Check sheet for the modelled part. Datum: model origin and axes. Units: mm. A direction names the side the tool comes from. Round coordinates to 2 decimals unless told otherwise and drop trailing zeros. Loops run counter-clockwise (first coordinate to the right, second up) from the corner with the lowest first, then second, coordinate; pieces in that order, holes last. Notation, with made-up numbers: (43, 16.5) -> (75, 16.5) arc R22 cw to (75, 38.5) -> close; hole circle Ø4 at (23.5, 61.5). An arc over 180 degrees is marked (long way). Use one line per item in the form item = value. Start each with the question number.
(1) Set-up check for faces 4 (the flat face through (150, 14, -71)), 5 (the flat face through (25, 4, -49.014)), 6 (the flat face through (191, 4, 9.986)), 7 (the flat face through (99, 8, 8)), 8 (the cylindrical face through (24, 4, 16)): record each of +Z, -Z, +X, -X, +Y, -Y from which the full face is reachable in a straight line by a thin tool's end or side.
(2) Sectioned sample at A-A (x = 127.5). Record the cut outline in (y, z).
(3) Sectioned sample at C-C (z = -15). Record the cut outline in (x, y).
(4) Sectioned sample at B-B (y = 14). Record the cut outline in (x, z).
(5) Draft check along Z on faces 1 (the cylindrical face through (99.3, 35.496, -77.588)), 2 (the flat face through (101, 18, -65)), 3 (the flat face through (9, 4, 9.986)). Enter one of: released by +Z, released by -Z, zero draft, split by the parting line, or undercut.
(6) Material ranges on probe 1 along Z at (x, y) = (9.5, 7.5); probe 2 along Z at (x, y) = (52, 18.5); probe 3 along Y at (x, z) = (136, -4.5), recorded low to high. Write a range as [from, to].
(7) Go/stop test with flat-tipped pins: pin 1 (8 mm diameter, centred on x = 113.5, y = 15.5, fed in from +Z); pin 2 (4 mm diameter, centred on x = 11.5, y = 3.5, fed in from -Z); pin 3 (10 mm diameter, centred on x = 60.5, z = -36.5, fed in from -Y); pin 4 (10 mm diameter, centred on x = 81.5, z = -54.5, fed in from +Y). Record where each tip stops, or that it passes through.
from build123d import *

# Parameters (mm, degrees)
EXTRUDE_1_DEPTH     = 200
SKETCH_2_W          = 50
SKETCH_2_H          = 30
CUT_EXTRUDE_1_DEPTH = 52
CUT_EXTRUDE_2_DEPTH = 10
CUT_EXTRUDE_4_DEPTH = 105.198677084


with BuildPart() as part:
    # Эскиз1 → Бобышка-Вытянуть1 (new body)
    with BuildSketch(Plane(origin=(0, 0, 0), x_dir=(0, 0, -1), z_dir=(1, 0, 0))):
        with BuildLine():
            Line((-80.986257223, 0), (79.013742777, 0))
            Line((79.013742777, 0), (79.013742777, 32))
            ThreePointArc((79.013742777, 32), (77.549276683, 35.535533906), (74.013742777, 37))
            Line((74.013742777, 37), (71.922596638, 37))
            ThreePointArc((71.922596638, 37), (69.613853571, 36.435054166), (67.826836416, 34.867882182))
            Line((67.826836416, 34.867882182), (49.013742777, 8))
            Line((49.013742777, 8), (-80.986257223, 8))
            Line((-80.986257223, 8), (-80.986257223, 0))
        make_face()
    extrude(amount=EXTRUDE_1_DEPTH)

    # Эскиз2 → Вырез-Вытянуть1 (cut)
    with BuildSketch(Plane.XZ):
        with Locations((25, -64.013742777)):
            Rectangle(SKETCH_2_W, SKETCH_2_H)
        with Locations((175, -64.013742777)):
            Rectangle(SKETCH_2_W, SKETCH_2_H)
    extrude(amount=-CUT_EXTRUDE_1_DEPTH, mode=Mode.SUBTRACT)

    # Эскиз3 → Вырез-Вытянуть2 (cut)
    with BuildSketch(Plane.XZ):
        with BuildLine():
            Line((18, 9.986257223), (0, 9.986257223))
            ThreePointArc((0, 9.986257223), (-6, 15.986257223), (0, 21.986257223))
            Line((0, 21.986257223), (18, 21.986257223))
            ThreePointArc((18, 21.986257223), (24, 15.986257223), (18, 9.986257223))
        make_face()
        with BuildLine():
            Line((182, 9.986257223), (200, 9.986257223))
            ThreePointArc((200, 9.986257223), (206, 15.986257223), (200, 21.986257223))
            Line((200, 21.986257223), (182, 21.986257223))
            ThreePointArc((182, 21.986257223), (176, 15.986257223), (182, 9.986257223))
        make_face()
    extrude(amount=-CUT_EXTRUDE_2_DEPTH, mode=Mode.SUBTRACT)

    # Эскиз4 → Вырез-Вытянуть4 (cut)
    with BuildSketch(Plane(origin=(150, 0, 0), x_dir=(0, 0, -1), z_dir=(1, 0, 0))):
        Polygon((67.577347999, 37), (67.577347999, 18), (62.577347999, 18), (62.577347999, 8), (49.013742777, 8), (49.013742777, 37), align=None)
    extrude(amount=-CUT_EXTRUDE_4_DEPTH, mode=Mode.SUBTRACT)


solid = part.part
Checks:
q1.face_4 = -Z, +X, +Y, -Y
q1.face_5 = -Z, -X, +Y, -Y
q1.face_6 = +X, +Y, -Y
q1.face_7 = +Z, +X, -X, +Y
q1.face_8 = -X, +Y, -Y
q2.outline = (0, -79.01) -> (32, -79.01) arc R5 ccw to (37, -74.01) -> (37, -71.92) arc R5 ccw to (34.87, -67.83) -> (34.51, -67.58) -> (18, -67.58) -> (18, -62.58) -> (8, -62.58) -> (8, 80.99) -> (0, 80.99) -> close
q3.outline = (0, 0) -> (200, 0) -> (200, 8) -> (0, 8) -> close
q4.outline = (50, -79.01) -> (150, -79.01) -> (150, -62.58) -> (50, -62.58) -> close
q5.face_1 = released by -Z
q5.face_2 = zero draft
q5.face_3 = undercut
q6.probe_1 = [-49.01, 9.99], [21.99, 80.99]
q6.probe_2 = [-79.01, -67.58]
q6.probe_3 = [0, 8]
q7.pin_1 = -62.58
q7.pin_2 = -49.01
q7.pin_3 = 0
q7.pin_4 = 8
